```python
from build123d import *

# Parameters (mm, degrees)
SKETCH1_W           = 5
SKETCH1_H           = 5
BOSS_EXTRUDE1_DEPTH = 270
SKETCH1_3_W         = 5
SKETCH1_3_H         = 10
CUT_EXTRUDE1_DEPTH  = 645
CIRPATTERN1_COUNT   = 4


with BuildPart() as part:
    # Sketch1 → Boss-Extrude1 (new body)
    with BuildSketch(Plane.XY):
        Polygon((-2.5, 10), (-10, 10), (-10, -10), (10, -10), (10, 10), (2.5, 10), (2.5, 5), (-2.5, 5), align=None)
        with Locations((0, 7.5)):
            Rectangle(SKETCH1_W, SKETCH1_H)
    extrude(amount=-BOSS_EXTRUDE1_DEPTH)

    # Sketch1_3 → Cut-Extrude1 (cut)
    with BuildSketch(Plane.XY):
        with Locations((0, 10)):
            Rectangle(SKETCH1_3_W, SKETCH1_3_H)
    cut_extrude1 = extrude(amount=-CUT_EXTRUDE1_DEPTH, mode=Mode.SUBTRACT)

    # CirPattern1: Cut-Extrude1 ×4 about axis
    cirpattern1_axis = Axis((0, 0, 0), (0, 0, 1))
    for i in range(1, CIRPATTERN1_COUNT):
        add(cut_extrude1.rotate(cirpattern1_axis, i * 360 / CIRPATTERN1_COUNT), mode=Mode.SUBTRACT)


solid = part.part
```
CAD build for the part. Positions are in the model's coordinates, mm. A direction names the side the tool comes from. Give positions to 0.01 mm unless a question says otherwise; leave off trailing zeros. Loops run counter-clockwise (first coordinate to the right, second up) from the corner with the lowest first, then second, coordinate; pieces in that order, holes last. Notation, with made-up numbers: (25.5, 13) -> (63.5, 13) arc R31 cw to (63.5, 39) -> close; hole circle Ø6 at (40, 54.5). An arc over 180 degrees is marked (long way). Use a Markdown table: item, result.
1. Which spindle directions (+Z, -Z, +X, -X, +Y, -Y) get a long thin tool onto all of the face, cutting with end or side? Do faces 1 (the flat face through (-2.5, 7, -133)), 2 (the flat face through (0, -5, -133)), 3 (the flat face through (-7, 2.5, -133)). Say none if no direction does.
Check result:
| item | result |
|---|---|
| face 1 | +Z, -Z, +Y |
| face 2 | +Z, -Z, -Y |
| face 3 | +Z, -Z, -X |
2. Wall check: L1, parallel to X at y = 8.5, z = -230; L2, parallel to X at y = 2.25, z = -69. Give the ranges that are in metal, low to high. Write a range as [from, to].
Check result:
| item | result |
|---|---|
| L1 | x = [-10, -2.5], [2.5, 10] |
| L2 | x = [-5, 5] |
3. Flat gauge pins, fed straight in: pin 1 (1.5 mm diameter, centred on y = 1, z = -136, fed in from +X); pin 2 (2 mm diameter, centred on x = -0.5, z = -76, fed in from +Y). Where does each tip first touch, or does it go through?
Check result:
| item | result |
|---|---|
| pin 1 | stops at x = 5 |
| pin 2 | stops at y = 5 |
4. Mould opens along Y. For faces 4 (the flat face through (7, 2.5, -133)), 5 (the flat face through (-6, 10, -133)), 6 (the flat face through (0, 0, -270)) say: pulls with the +Y half, pulls with the -Y half, needs draft (parallel to the pull), parting line crosses it, or undercut.
Check result:
| item | result |
|---|---|
| face 4 | undercut |
| face 5 | pulls with the +Y half |
| face 6 | needs draft |
5. Slice it at A-A (y = -7.5). List the corners of the cut face in (x, z), plus the area to 3 significant figures.
Check result:
| item | result |
|---|---|
| outline | (-10, -270) -> (-2.5, -270) -> (-2.5, 0) -> (-10, 0) -> close; (2.5, -270) -> (10, -270) -> (10, 0) -> (2.5, 0) -> close |
| area | 4,050 mm^2 |
6. Slice it at B-B (z = -41). List the corners of the cut face in (x, y).
Check result:
| item | result |
|---|---|
| outline | (-10, -10) -> (-2.5, -10) -> (-2.5, -5) -> (2.5, -5) -> (2.5, -10) -> (10, -10) -> (10, -2.5) -> (5, -2.5) -> (5, 2.5) -> (10, 2.5) -> (10, 10) -> (2.5, 10) -> (2.5, 5) -> (-2.5, 5) -> (-2.5, 10) -> (-10, 10) -> (-10, 2.5) -> (-5, 2.5) -> (-5, -2.5) -> (-10, -2.5) -> close |
